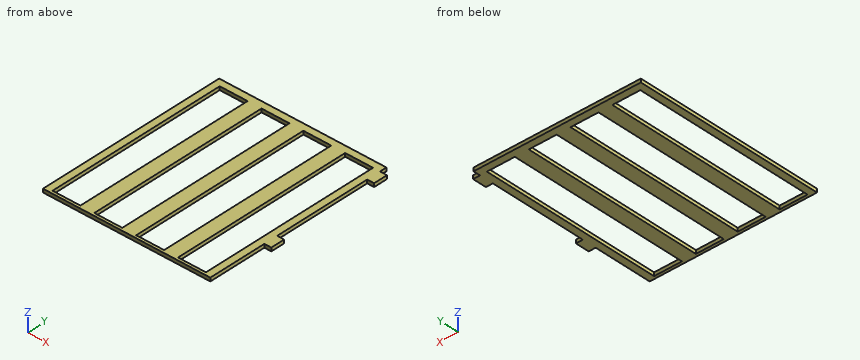
Autodesk Inventor part; units mm, degrees
ref_plane "YZ Plane" through (0, 0, 0) normal (1, 0, 0) x (0, 1, 0)
ref_plane "XZ Plane" through (0, 0, 0) normal (0, 1, 0) x (-1, 0, 0)
ref_plane "XY Plane" through (0, 0, 0) normal (0, 0, 1) x (1, 0, 0)
sketch "Sketch1" plane through (0, 0, 0) normal (0, 0, 1) x (1, 0, 0)
  line L0 (0, 0) -> (0, 177.8)
  line L1 (0, 177.8) -> (152.4, 177.8)
  line L2 (152.4, 177.8) -> (152.4, 0)
  line L3 (152.4, 0) -> (0, 0)
  dimension "d0" = 177.8
  dimension "d1" = 152.4
extrude "Extrusion1" add sketch "Sketch1" along normal blind 3.175
sketch "Sketch2" plane through (0, 0, 0) normal (0, 0, -1) x (-1, 0, 0)
  line L0 (-152.4, 177.8) -> (0, 177.8)
  line L1 (-152.4, 0) -> (-152.4, 177.8)
  line L2 (0, 0) -> (-152.4, 0)
  line L3 (-152.4, 171.45) -> (-158.75, 171.45)
  line L4 (-158.75, 171.45) -> (-158.75, 158.75)
  line L5 (-158.75, 158.75) -> (-152.4, 158.75)
  line L6 (-152.4, 69.85) -> (-158.75, 69.85)
  line L7 (-158.75, 69.85) -> (-158.75, 57.15)
  line L8 (-158.75, 57.15) -> (-152.4, 57.15)
  dimension "d9" = 6.35
  dimension "d10" = 12.7
  dimension "d11" = 6.35
  dimension "d12" = 12.7
  dimension "d13" = 88.9
  dimension "d14" = 6.35
extrude "Extrusion2" add sketch "Sketch2" against normal blind 3.175
sketch "Sketch3" plane through (0, 0, 0) normal (0, 0, -1) x (-1, 0, 0)
  line L0 (-152.4, 177.8) -> (0, 177.8)
  line L1 (-152.4, 171.45) -> (-152.4, 177.8)
  line L2 (0, 0) -> (-152.4, 0)
  line L3 (-146.05, 171.45) -> (-120.65, 171.45)
  line L4 (-120.65, 171.45) -> (-120.65, 6.35)
  line L5 (-120.65, 6.35) -> (-146.05, 6.35)
  line L6 (-146.05, 171.45) -> (-146.05, 6.35)
  line L7 (-107.95, 171.45) -> (-82.55, 171.45)
  line L8 (-82.55, 171.45) -> (-82.55, 6.35)
  line L9 (-82.55, 6.35) -> (-107.95, 6.35)
  line L10 (-107.95, 171.45) -> (-107.95, 6.35)
  line L11 (-69.85, 171.45) -> (-44.45, 171.45)
  line L12 (-44.45, 171.45) -> (-44.45, 6.35)
  line L13 (-44.45, 6.35) -> (-69.85, 6.35)
  line L14 (-69.85, 171.45) -> (-69.85, 6.35)
  line L15 (-31.75, 171.45) -> (-6.35, 171.45)
  line L16 (-6.35, 171.45) -> (-6.35, 6.35)
  line L17 (-6.35, 6.35) -> (-31.75, 6.35)
  line L18 (-31.75, 171.45) -> (-31.75, 6.35)
  dimension "d17" = 25.4
  dimension "d18" = 25.4
  dimension "d20" = 6.35
  dimension "d21" = 6.35
  dimension "d22" = 6.35
  dimension "d25" = 38.1
extrude "Extrusion3" cut sketch "Sketch3" against normal blind 3.175
sketch "Sketch4" plane through (0, 0, 0) normal (0, 0, -1) x (-1, 0, 0)
  line L0 (0, 177.8) -> (0, 0)
  line L1 (-152.4, 0) -> (-152.4, 57.15)
  line L2 (0, 0) -> (-152.4, 0)
  line L3 (-152.4, 3.81) -> (0, 3.81)
  dimension "d32" = 3.81
extrude "Extrusion4" cut sketch "Sketch4" against normal blind 25.4
properties part number "Backboard" material "Polycarbonate, Clear"
Geometry: final body of the model. Coordinates: model frame, mm. Give positions to 0.01 mm unless a question says otherwise; leave off trailing zeros. Write each loop counter-clockwise with the first axis right and the second up, starting at its lowest first coordinate (ties: lowest second). Pieces come first, ordered by that corner, then holes.
1. Section query D-D, the plane y = 148. Return loops of the section in (x, z) (3 decimals), then the cut area to 3 significant figures.
2. Section query B-B, the plane y = 60. Return loops of the section in (x, z) (3 decimals).
3. Section query A-A, the plane z = 2.4. Return loops of the section in (x, y), then the cut area to 3 significant figures.
4. Pin query (flat end, axial travel): P1, Ø1.6, axis at y = 93, z = 2, coming from the +X side. Return the tip coordinate at first contact, or that it passes through.
5. Section query C-C, the plane x = 49. Return loops of the section in (y, z) (3 decimals).
6. Line query: probe 1 along X at (y, z) = (23, 1.6); probe 2 along X at (y, z) = (169.5, 2.45); probe 3 along Y at (x, z) = (97.5, 2.05). Output: solid intervals per line, ascending.
Computed:
1. outline: (0, 0) - (6.35, 0) - (6.35, 3.175) - (0, 3.175) - close; (31.75, 0) - (44.45, 0) - (44.45, 3.175) - (31.75, 3.175) - close; (69.85, 0) - (82.55, 0) - (82.55, 3.175) - (69.85, 3.175) - close; (107.95, 0) - (120.65, 0) - (120.65, 3.175) - (107.95, 3.175) - close; (146.05, 0) - (152.4, 0) - (152.4, 3.175) - (146.05, 3.175) - close
1. area: 161 mm2
2. outline: (0, 0) - (6.35, 0) - (6.35, 3.175) - (0, 3.175) - close; (31.75, 0) - (44.45, 0) - (44.45, 3.175) - (31.75, 3.175) - close; (69.85, 0) - (82.55, 0) - (82.55, 3.175) - (69.85, 3.175) - close; (107.95, 0) - (120.65, 0) - (120.65, 3.175) - (107.95, 3.175) - close; (146.05, 0) - (158.75, 0) - (158.75, 3.175) - (146.05, 3.175) - close
3. outline: (0, 3.81) - (152.4, 3.81) - (152.4, 57.15) - (158.75, 57.15) - (158.75, 69.85) - (152.4, 69.85) - (152.4, 158.75) - (158.75, 158.75) - (158.75, 171.45) - (152.4, 171.45) - (152.4, 177.8) - (0, 177.8) - close; hole (6.35, 6.35) - (31.75, 6.35) - (31.75, 171.45) - (6.35, 171.45) - close; hole (44.45, 6.35) - (69.85, 6.35) - (69.85, 171.45) - (44.45, 171.45) - close; hole (82.55, 6.35) - (107.95, 6.35) - (107.95, 171.45) - (82.55, 171.45) - close; hole (120.65, 6.35) - (146.05, 6.35) - (146.05, 171.45) - (120.65, 171.45) - close
3. area: 9,900 mm2
4. P1: stops at x = 152.4
5. outline: (3.81, 0) - (6.35, 0) - (6.35, 3.175) - (3.81, 3.175) - close; (171.45, 0) - (177.8, 0) - (177.8, 3.175) - (171.45, 3.175) - close
6. probe 1: x = 0 to 6.35, 31.75 to 44.45, 69.85 to 82.55, 107.95 to 120.65, 146.05 to 152.4
6. probe 2: x = 0 to 6.35, 31.75 to 44.45, 69.85 to 82.55, 107.95 to 120.65, 146.05 to 158.75
6. probe 3: y = 3.81 to 6.35, 171.45 to 177.8
